Could you check a few things on this model? Use its own coordinates, in mm. Face numbers are marked on the shaded views. A direction names the side the tool comes from. Give positions to 0.01 mm unless a question says otherwise; leave off trailing zeros. Loops run counter-clockwise (first coordinate to the right, second up) from the corner with the lowest first, then second, coordinate; pieces in that order, holes last.
1. Thinking about a two-plate mould opening in Y: for the marked faces 1, 2, 3 and 4, which applies, +Y half, -Y half, draft (parallel to the pull), parting line (faces both ways), or undercut?
2. For the marked faces 5 and 6, which set-ups out of +Z, -Z, +X, -X, +Y, -Y let a thin tool reach every point of the face, with its end or its side?
3. Imagine slicing it at B-B (y = 0). List the corners of the cut face in (x, z) for me (1 decimal).
4. Imagine slicing it at D-D (x = 5.5). List the corners of the cut face in (y, z) for me (3 decimals), plus the area to 3 significant figures.
5. Imagine slicing it at C-C (z = -9.5). List the corners of the cut face in (x, y) for me (3 decimals).
6. For P1, Ø10, axis at x = 0, y = 0, coming from the -Z side, with a flat end and sliding along its axis, tell me the tip position at first contact or that it passes through.
7. I need wall thicknesses on line 1 along Y through (x, z) = (0, -0.6); line 2 along Y through (x, z) = (0, -5.35); line 3 along X through (y, z) = (3, -9.25) (3 decimals). Which ranges of each line are inside material? Lowest first, please.
```python
from build123d import *

# Parameters (mm, degrees)
F0_W     = 30.12
F0_H     = 22.5
F1_DEPTH = 11.407
F2_W     = 19.53
F2_H     = 11.91
F3_DEPTH = 4.71
F4_R     = 4.1275
F5_DEPTH = 1.905
F6_R     = 3.05689
F7_DEPTH = 6.0706


with BuildPart() as f1:
    # F0 (on Top) → F1 (new body)
    with BuildSketch(Plane.XY):
        Rectangle(F0_W, F0_H)
    extrude(amount=-F1_DEPTH)

    # F2 (on face) → F3 (cut)
    with BuildSketch(Plane(origin=(0, 0, -11.407), x_dir=(1, 0, 0), z_dir=(0, 0, -1))):
        Rectangle(F2_W, F2_H)
    extrude(amount=-F3_DEPTH, mode=Mode.SUBTRACT)

    # F4 (on face) → F5 (cut)
    with BuildSketch(Plane.XY):
        Circle(F4_R)
    extrude(amount=-F5_DEPTH, mode=Mode.SUBTRACT)

    # F6 (on face) → F7 (cut)
    with BuildSketch(Plane.XY.offset(-1.905)):
        Circle(F6_R)
    extrude(amount=-F7_DEPTH, mode=Mode.SUBTRACT)


solid = f1.part
```
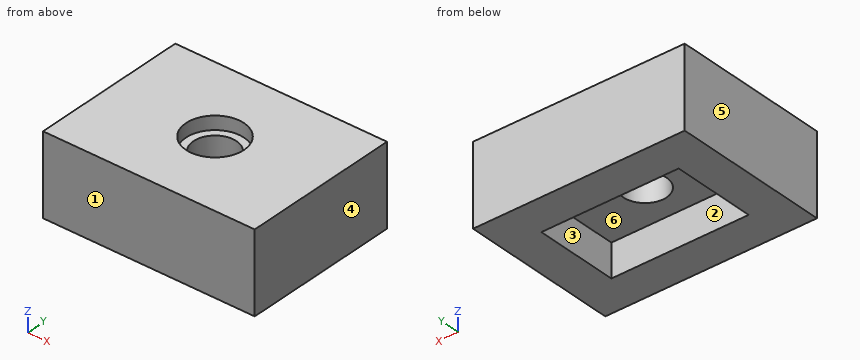
Derived:
1. face 1: -Y half
1. face 2: undercut
1. face 3: undercut
1. face 4: draft
2. face 5: +Z, -Z, -X, +Y, -Y
2. face 6: -Z
3. outline: (-15.1, -11.4) - (-9.8, -11.4) - (-9.8, -6.7) - (-3.1, -6.7) - (-3.1, -1.9) - (-4.1, -1.9) - (-4.1, 0) - (-15.1, 0) - close; (3.1, -6.7) - (9.8, -6.7) - (9.8, -11.4) - (15.1, -11.4) - (15.1, 0) - (4.1, 0) - (4.1, -1.9) - (3.1, -1.9) - close
4. outline: (-11.25, -11.407) - (-5.955, -11.407) - (-5.955, -6.697) - (5.955, -6.697) - (5.955, -11.407) - (11.25, -11.407) - (11.25, 0) - (-11.25, 0) - close
4. area: 201 mm2
5. outline: (-15.06, -11.25) - (15.06, -11.25) - (15.06, 11.25) - (-15.06, 11.25) - close; hole (-9.765, -5.955) - (9.765, -5.955) - (9.765, 5.955) - (-9.765, 5.955) - close
6. P1: stops at z = -6.7
7. line 1: y = -11.25 to -4.13, 4.13 to 11.25
7. line 2: y = -11.25 to -3.06, 3.06 to 11.25
7. line 3: x = -15.06 to -9.765, 9.765 to 15.06
